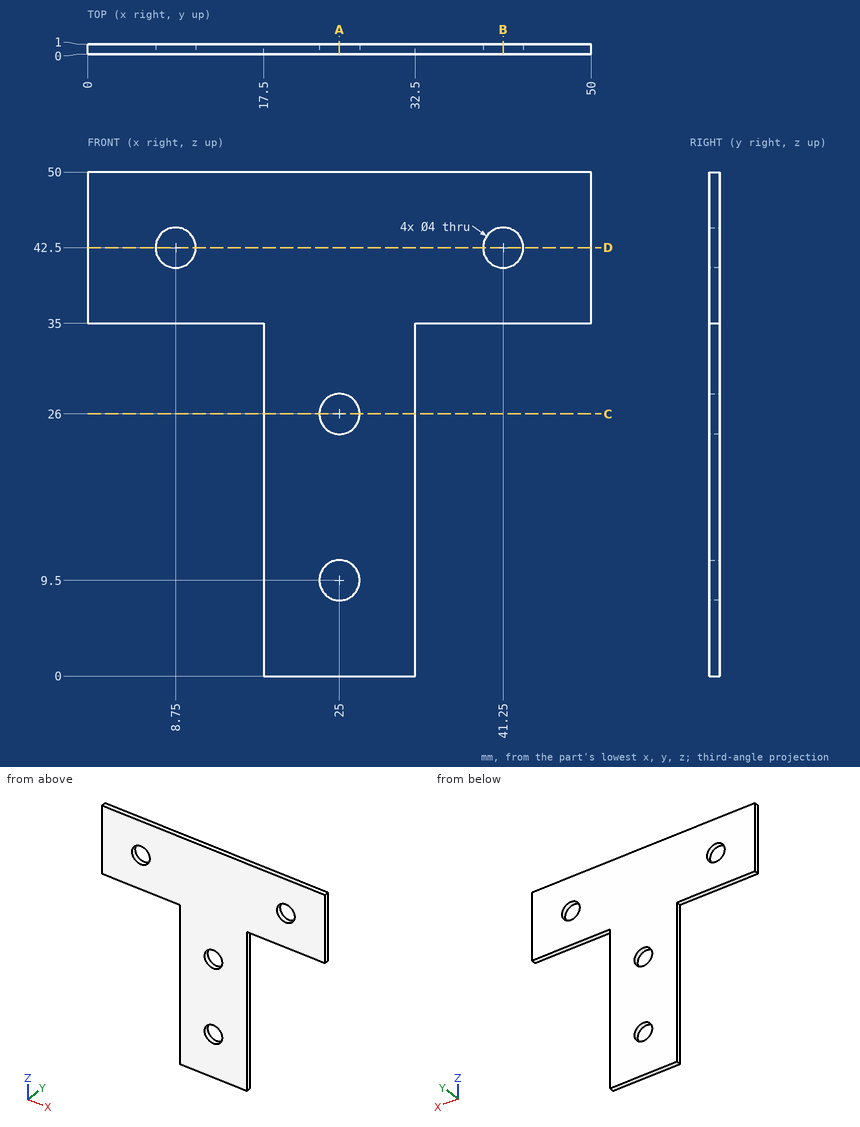
Answer from the drawing. Dimensions are ordinates in mm from the lowest x, y and z of the part. Give positions to 0.01 mm unless a question says otherwise; leave off trailing zeros. Loops run counter-clockwise (first coordinate to the right, second up) from the corner with the lowest first, then second, coordinate; pieces in that order, holes last. Notation, with made-up numbers: (25.25, 81) - (68.25, 81) arc R13 ccw to (68.25, 104) - close; hole circle Ø8 at (19, -4.75). An arc over 180 degrees is marked (long way). Answer as a JSON object with one key per item and string values.
1. A cutting plane is placed at B-B (x = 41.25). Write down the section's boundary in (y, z), then the cut area to 3 significant figures.
Determined:
{"outline": "(0, 35) - (1, 35) - (1, 40.5) - (0, 40.5) - close; (0, 44.5) - (1, 44.5) - (1, 50) - (0, 50) - close", "area": "11.0 mm²"}
2. A cutting plane is placed at D-D (z = 42.5). Write down the section's boundary in (x, y).
Determined:
{"outline": "(0, 0) - (6.75, 0) - (6.75, 1) - (0, 1) - close; (10.75, 0) - (39.25, 0) - (39.25, 1) - (10.75, 1) - close; (43.25, 0) - (50, 0) - (50, 1) - (43.25, 1) - close"}
3. A cutting plane is placed at C-C (z = 26). Write down the section's boundary in (x, y).
Determined:
{"outline": "(17.5, 0) - (23, 0) - (23, 1) - (17.5, 1) - close; (27, 0) - (32.5, 0) - (32.5, 1) - (27, 1) - close"}
4. Find the intervals of material crossed by L1, parallel to Z at x = 25, y = 0.3; L2, parallel to Z at x = 8.75, y = 0.5; L3, parallel to X at y = 0.55, z = 9.5, in increasing order. Write a range as [from, to].
Determined:
{"L1": "[0, 7.5], [11.5, 24], [28, 50]", "L2": "[35, 40.5], [44.5, 50]", "L3": "[17.5, 23], [27, 32.5]"}
5. A flat-ended cylindrical pin translates along its axis: pin 1 Ø6.5 at (x, z) = (8.75, 42.5) entering from +Y. Find the tip coordinate at first contact, or state that the pin passes through.
Determined:
{"pin 1": "y = 1"}
6. A cutting plane is placed at A-A (x = 25). Write down the section's boundary in (y, z), then the cut area to 3 significant figures.
Determined:
{"outline": "(0, 0) - (1, 0) - (1, 7.5) - (0, 7.5) - close; (0, 11.5) - (1, 11.5) - (1, 24) - (0, 24) - close; (0, 28) - (1, 28) - (1, 50) - (0, 50) - close", "area": "42.0 mm²"}
